Autodesk Inventor part; units mm, degrees
ref_plane "YZ Plane" through (0, 0, 0) normal (1, 0, 0) x (0, 1, 0)
ref_plane "XZ Plane" through (0, 0, 0) normal (0, 1, 0) x (-1, 0, 0)
ref_plane "XY Plane" through (0, 0, 0) normal (0, 0, 1) x (1, 0, 0)
sketch "Skizze1" plane through (0, 0, 0) normal (0, 1, 0) x (-1, 0, 0)
  line L0 (-15, 15) -> (15, 15)
  line L1 (15, 15) -> (15, -15)
  line L2 (15, -15) -> (-15, -15)
  line L3 (-15, -15) -> (-15, 15)
  line L4 (-15, 15) -> (15, -15) construction
  line L5 (15, 15) -> (-15, -15) construction
  point P0 (0, 0)
  dimension "d0" = 30
  dimension "d1" = 30
extrude "Extrusion1" add sketch "Skizze1" along normal blind 15
sketch "Skizze2" plane through (-15, 0, 15) normal (0, 0, 1) x (1, 0, 0)
  circle A0 centre (15, 0) radius 0.8
  dimension "d4" = 1.6
hole "Bohrung1" at (0, 0, 15) direction (0, 0, -1) diameter 1.6 end through all
sketch "Skizze3" plane through (0, 15, 0) normal (0, 1, 0) x (1, 0, 0)
  point P0 (0, 0)
hole "Bohrung2" at (0, 15, 0) direction (0, -1, 0) diameter 0.8 end through all
sketch "Skizze4" plane through (0, 15, 0) normal (0, 1, 0) x (1, 0, 0)
  point P0 (0, 0)
  point P1 (0, 0)
hole "Bohrung3" at (0, 15, 0) direction (0, -1, 0) diameter 5.5 depth 5.7
sketch "Skizze5" plane through (0, 15, 0) normal (0, 1, 0) x (1, 0, 0)
  point P0 (0, 0)
sketch "Skizze6" plane through (0, 15, 0) normal (0, 1, 0) x (1, 0, 0)
  line L0 (10.5, 10.5) -> (-10.5, 10.5)
  line L1 (-10.5, 10.5) -> (-10.5, -10.5)
  line L2 (-10.5, -10.5) -> (10.5, -10.5)
  line L3 (10.5, -10.5) -> (10.5, 10.5)
  circle A0 centre (0, 0) radius 0.4
  line L4 (10.5, 10.5) -> (-10.5, -10.5) construction
  line L5 (-10.5, 10.5) -> (10.5, -10.5) construction
  dimension "d26" = 21
  dimension "d27" = 21
hole "Bohrung4" at (10.5, 15, 10.5) at (-10.5, 15, 10.5) at (-10.5, 15, -10.5) at (10.5, 15, -10.5) direction (0, -1, 0) diameter 3 end through all
properties part number "LS1_Aufsatz" material "PMMA-Kunststoff"
Check sheet for the modelled part. Datum: model origin and axes. Units: mm. A direction names the side the tool comes from. Coordinates: 2 decimals unless noted, no trailing zeros. Loops run counter-clockwise (first coordinate to the right, second up) from the corner with the lowest first, then second, coordinate; pieces in that order, holes last. Notation, with made-up numbers: (67, -2) -> (119, -2) arc R24 ccw to (119, 28) -> close; hole circle Ø1 at (-8.5, 32). An arc over 180 degrees is marked (long way). Answer in a Markdown table with one row per item.
1. Sectioned sample at A-A, the plane x = 0. Record the boundary of the cut face in (y, z), then the cut area to 3 significant figures.
Check values:
| item | result |
|---|---|
| outline | (0.8, -15) -> (15, -15) -> (15, -2.75) -> (9.3, -2.75) -> (9.3, -0.4) -> (0.8, -0.4) -> close; (0.8, 0.4) -> (9.3, 0.4) -> (9.3, 2.75) -> (15, 2.75) -> (15, 15) -> (0.8, 15) -> close |
| area | 388 mm2 |
2. Sectioned sample at C-C, the plane z = 10.5. Record the boundary of the cut face in (x, y).
Check values:
| item | result |
|---|---|
| outline | (-15, 0) -> (-12, 0) -> (-12, 15) -> (-15, 15) -> close; (-9, 0) -> (-0.8, 0) arc R0.8 cw to (0.8, 0) -> (9, 0) -> (9, 15) -> (-9, 15) -> close; (12, 0) -> (15, 0) -> (15, 15) -> (12, 15) -> close |
3. Access from +Z, -Z, +X, -X, +Y, -Y to the whole of each face (thin tool, end or side, straight path). Record for faces 1 (the face through (1, 9.3, 0)), 2 (the face through (0, 7, -15)).
Check values:
| item | result |
|---|---|
| face 1 | +Y |
| face 2 | -Z, +X, -X, +Y, -Y |
4. Go/stop test with a flat-tipped pin: pin 1 (1.6 mm diameter, centred on x = -1, z = -1, fed in from +Y). Record where the tip stops, or that it passes through.
Check values:
| item | result |
|---|---|
| pin 1 | stops at y = 9.3 |
5. Release check for a two-part mould opening along Z. For faces 3 (the face through (4, 15, 0)), 4 (the face through (11.4, 7.4, -11.7)), 5 (the face through (-10.57, 7.4, -12)), 6 (the face through (0, 7, 15)) record: released by +Z, released by -Z, zero draft, split by the parting line, or undercut.
Check values:
| item | result |
|---|---|
| face 3 | zero draft |
| face 4 | undercut |
| face 5 | undercut |
| face 6 | released by +Z |
6. Sectioned sample at B-B, the plane y = 10.75. Record the boundary of the cut face in (x, z), then the cut area to 3 significant figures.
Check values:
| item | result |
|---|---|
| outline | (-15, -15) -> (15, -15) -> (15, 15) -> (-15, 15) -> close; hole circle Ø3 at (-10.5, -10.5); hole circle Ø3 at (-10.5, 10.5); hole circle Ø5.5 at (0, 0); hole circle Ø3 at (10.5, -10.5); hole circle Ø3 at (10.5, 10.5) |
| area | 848 mm2 |
7. Material ranges on line 1 along X through (y, z) = (4.25, -10.5); line 2 along X through (y, z) = (13.2, 0), recorded low to high. Write a range as [from, to].
Check values:
| item | result |
|---|---|
| line 1 | x = [-15, -12], [-9, 9], [12, 15] |
| line 2 | x = [-15, -2.75], [2.75, 15] |
8. Sectioned sample at D-D, the plane x = -10.5. Record the boundary of the cut face in (y, z), then the cut area to 3 significant figures.
Check values:
| item | result |
|---|---|
| outline | (0, -15) -> (15, -15) -> (15, -12) -> (0, -12) -> close; (0, -9) -> (15, -9) -> (15, 9) -> (0, 9) -> close; (0, 12) -> (15, 12) -> (15, 15) -> (0, 15) -> close |
| area | 360 mm2 |
